Read the model definition and answer for the solid it produces. Units are mm, in the model's axes. A direction names the side the tool comes from. Give positions to 0.01 mm unless a question says otherwise; leave off trailing zeros. Write each loop counter-clockwise with the first axis right and the second up, starting at its lowest first coordinate (ties: lowest second). Pieces come first, ordered by that corner, then holes.
```python
from build123d import *

# Parameters (mm, degrees)
SKETCH_2_W           = 32.3
SKETCH_2_H           = 12.2
SKETCH_2_R           = 1
EXTRUDE_1_DEPTH      = 2.4
EXTRUDE_2_DEPTH      = 16.3
EXTRUDE_2_DEPTH_BACK = 6.9
SKETCH_3_W           = 22.5
SKETCH_3_H           = 12.2


with BuildPart() as part:
    # 草圖2 → 填料-伸長1 (new body)
    with BuildSketch(Plane(origin=(0, 0, 0), x_dir=(1, 0, 0), z_dir=(0, 1, 0))):
        Rectangle(SKETCH_2_W, SKETCH_2_H)
        with Locations(Location((-13.75, 0, 0), (0, 0, 270))):
            Circle(SKETCH_2_R, mode=Mode.SUBTRACT)
        with Locations(Location((13.75, 0, 0), (0, 0, 270))):
            Circle(SKETCH_2_R, mode=Mode.SUBTRACT)
    extrude(amount=EXTRUDE_1_DEPTH)

    # 草圖3 → 填料-伸長2 (add, two sides: drawn at the far end of the back side and taken through both)
    with BuildSketch(Plane.XZ.offset(-EXTRUDE_2_DEPTH_BACK)):
        Rectangle(SKETCH_3_W, SKETCH_3_H)
    extrude(amount=EXTRUDE_2_DEPTH + EXTRUDE_2_DEPTH_BACK)


solid = part.part
```
Item 1: Section A-A (z = 0) is taken. Write down the section's boundary in (x, y), and give its area (3 significant figures).
Result set:
outline: (-16.15, 0) - (-14.75, 0) - (-14.75, 2.4) - (-16.15, 2.4) - close; (-12.75, 0) - (-11.25, 0) - (-11.25, -16.3) - (11.25, -16.3) - (11.25, 0) - (12.75, 0) - (12.75, 2.4) - (11.25, 2.4) - (11.25, 6.9) - (-11.25, 6.9) - (-11.25, 2.4) - (-12.75, 2.4) - close; (14.75, 0) - (16.15, 0) - (16.15, 2.4) - (14.75, 2.4) - close
area: 536 mm2
Item 2: Which of the six approach directions +Z, -Z, +X, -X, +Y, -Y give full straight-line access (tool end or side, diameter ignored) to faces 5 (the flat face through (15, 0, 0)), 6 (the flat face through (15, 2.4, 0)), 7 (the flat face through (-11.25, -8, 0))?
Result set:
face 5: +Z, -Z, +X, -Y
face 6: +Z, -Z, +X, +Y
face 7: +Z, -Z, -X, -Y
Item 3: Each of these flat-tipped pins is pushed along its axis until it touches: pin 1 Ø2.5 at (x, z) = (-13.5, -1) entering from +Y; pin 2 Ø10 at (x, y) = (-12.5, -10.5) entering from -Z; pin 3 Ø2 at (y, z) = (4, 1.5) entering from +X; pin 4 Ø3 at (x, z) = (-13.75, 0) entering from -Y. Where does it stop, or does it pass through?
Result set:
pin 1: stops at y = 2.4
pin 2: stops at z = -6.1
pin 3: stops at x = 11.25
pin 4: stops at y = 0
Item 4: Section D-D (z = 1.5) is taken. Write down the section's boundary in (x, y), and give its area (3 significant figures).
Result set:
outline: (-16.15, 0) - (-11.25, 0) - (-11.25, -16.3) - (11.25, -16.3) - (11.25, 0) - (16.15, 0) - (16.15, 2.4) - (11.25, 2.4) - (11.25, 6.9) - (-11.25, 6.9) - (-11.25, 2.4) - (-16.15, 2.4) - close
area: 546 mm2
Item 5: Determine the mould class of faces 1 (the flat face through (0, -5, 6.1)), 2 (the cylindrical face through (12.774, 1.183, -0.217)), 3 (the flat face through (0, -16.3, 0)), 4 (the cylindrical face through (-14.726, 1.183, -0.217)) for opening direction Z: pulls with the +Z half, pulls with the -Z half, needs draft (parallel to the pull), parting line crosses it, or undercut.
Result set:
face 1: pulls with the +Z half
face 2: undercut
face 3: needs draft
face 4: undercut
Item 6: Section C-C (x = 13.75) is taken. Write down the section's boundary in (y, z), and give its area (3 significant figures).
Result set:
outline: (0, -6.1) - (2.4, -6.1) - (2.4, -1) - (0, -1) - close; (0, 1) - (2.4, 1) - (2.4, 6.1) - (0, 6.1) - close
area: 24.5 mm2
Item 7: Section B-B (y = 1.75) is taken. Write down the section's boundary in (x, z), and give its area (3 significant figures).
Result set:
outline: (-16.15, -6.1) - (16.15, -6.1) - (16.15, 6.1) - (-16.15, 6.1) - close; hole circle Ø2 at (-13.75, 0); hole circle Ø2 at (13.75, 0)
area: 388 mm2
Item 8: Find the intervals of material crossed by line 1 along X through (y, z) = (1.05, 0); line 2 along X through (y, z) = (1.5, 0.75); line 3 along X through (y, z) = (3, 1), in increasing order.
Result set:
line 1: x = -16.15 to -14.75, -12.75 to 12.75, 14.75 to 16.15
line 2: x = -16.15 to -14.41, -13.09 to 13.09, 14.41 to 16.15
line 3: x = -11.25 to 11.25
